Work out the finished part from the listing and answer in its coordinate system (mm). A direction names the side the tool comes from. Give positions to 0.01 mm unless a question says otherwise; leave off trailing zeros. Loops run counter-clockwise (first coordinate to the right, second up) from the corner with the lowest first, then second, coordinate; pieces in that order, holes last. Notation, with made-up numbers: (61.25, -3.5) - (115.25, -3.5) arc R25 ccw to (115.25, 8.5) - close; hole circle Ø9 at (40.25, 45). An arc over 180 degrees is marked (long way). One line per item, written item: value.
from build123d import *

# Parameters (mm, degrees)
SKETCH1_W           = 228.6
SKETCH1_H           = 339.725
BOSS_EXTRUDE1_DEPTH = 6.35
SKETCH2_W           = 6.35
SKETCH2_H           = 19.05
BOSS_EXTRUDE2_DEPTH = 25.4
FILLET1_R           = 9.525
FILLET2_R           = 8
SKETCH3_R           = 4.7625
CUT_EXTRUDE1_DEPTH  = 401.415210282
SKETCH5_R           = 3.175
CUT_EXTRUDE2_DEPTH  = 411.263568484
SKETCH9_W           = 145.328
SKETCH9_H           = 196.09
CUT_EXTRUDE3_DEPTH  = 411.263568484
FILLET3_R           = 25.4
FILLET4_R           = 6.35


with BuildPart() as part:
    # Sketch1 → Boss-Extrude1 (new body)
    with BuildSketch(Plane.XY):
        with Locations((114.3, -169.8625)):
            Rectangle(SKETCH1_W, SKETCH1_H)
    extrude(amount=BOSS_EXTRUDE1_DEPTH)

    # Sketch2 → Boss-Extrude2 (add)
    with BuildSketch(Plane.XY.offset(6.35)):
        with Locations((22.225, -35.56)):
            Rectangle(SKETCH2_W, SKETCH2_H)
        with Locations((47.879, -35.56)):
            Rectangle(SKETCH2_W, SKETCH2_H)
        with Locations((149.479, -35.56)):
            Rectangle(SKETCH2_W, SKETCH2_H)
        with Locations((175.133, -35.56)):
            Rectangle(SKETCH2_W, SKETCH2_H)
        with Locations((22.225, -304.8)):
            Rectangle(SKETCH2_W, SKETCH2_H)
        with Locations((47.879, -304.8)):
            Rectangle(SKETCH2_W, SKETCH2_H)
        with Locations((149.479, -304.8)):
            Rectangle(SKETCH2_W, SKETCH2_H)
        with Locations((175.133, -304.8)):
            Rectangle(SKETCH2_W, SKETCH2_H)
        with Locations((175.553, -132.588)):
            Rectangle(SKETCH2_W, SKETCH2_H)
        with Locations((206.287, -132.588)):
            Rectangle(SKETCH2_W, SKETCH2_H)
    extrude(amount=BOSS_EXTRUDE2_DEPTH)

    # Fillet1
    fillet1_edges = [part.edges().sort_by_distance(p)[0] for p in [
        (22.225, -314.325, 31.75),
        (22.225, -295.275, 31.75),
        (47.879, -314.325, 31.75),
        (47.879, -295.275, 31.75),
        (149.479, -314.325, 31.75),
        (149.479, -295.275, 31.75),
        (175.133, -314.325, 31.75),
        (175.133, -295.275, 31.75),
        (206.287, -142.113, 31.75),
        (206.287, -123.063, 31.75),
        (175.553, -142.113, 31.75),
        (175.553, -123.063, 31.75),
        (175.133, -45.085, 31.75),
        (175.133, -26.035, 31.75),
        (149.479, -45.085, 31.75),
        (149.479, -26.035, 31.75),
        (47.879, -45.085, 31.75),
        (47.879, -26.035, 31.75),
        (22.225, -45.085, 31.75),
        (22.225, -26.035, 31.75),
    ]]
    fillet(fillet1_edges, radius=FILLET1_R - 0.0001)  # a hair under: the kernel refuses the full size

    # Fillet2
    fillet2_edges = [part.edges().sort_by_distance(p)[0] for p in [
        (22.225, -295.275, 6.35),
        (19.05, -304.8, 6.35),
        (25.4, -304.8, 6.35),
        (22.225, -314.325, 6.35),
        (44.704, -304.8, 6.35),
        (47.879, -314.325, 6.35),
        (51.054, -304.8, 6.35),
        (47.879, -295.275, 6.35),
        (22.225, -26.035, 6.35),
        (19.05, -35.56, 6.35),
        (25.4, -35.56, 6.35),
        (22.225, -45.085, 6.35),
        (44.704, -35.56, 6.35),
        (47.879, -45.085, 6.35),
        (51.054, -35.56, 6.35),
        (47.879, -26.035, 6.35),
        (149.479, -26.035, 6.35),
        (146.304, -35.56, 6.35),
        (152.654, -35.56, 6.35),
        (149.479, -45.085, 6.35),
        (171.958, -35.56, 6.35),
        (175.133, -45.085, 6.35),
        (178.308, -35.56, 6.35),
        (175.133, -26.035, 6.35),
        (175.553, -123.063, 6.35),
        (172.378, -132.588, 6.35),
        (178.728, -132.588, 6.35),
        (175.553, -142.113, 6.35),
        (203.112, -132.588, 6.35),
        (206.287, -142.113, 6.35),
        (209.462, -132.588, 6.35),
        (206.287, -123.063, 6.35),
        (171.958, -304.8, 6.35),
        (175.133, -314.325, 6.35),
        (178.308, -304.8, 6.35),
        (175.133, -295.275, 6.35),
        (149.479, -295.275, 6.35),
        (146.304, -304.8, 6.35),
        (152.654, -304.8, 6.35),
        (149.479, -314.325, 6.35),
    ]]
    fillet(fillet2_edges, radius=FILLET2_R)

    # Sketch3 → Cut-Extrude1 (cut, through all)
    with BuildSketch(Plane.ZY.offset(-19.05)):
        with Locations(Location((22.225, -35.56, 0), (0, 0, 180))):
            Circle(SKETCH3_R)
        with Locations(Location((22.225, -132.588, 0), (0, 0, 180))):
            Circle(SKETCH3_R)
        with Locations(Location((22.225, -304.8, 0), (0, 0, 180))):
            Circle(SKETCH3_R)
    extrude(amount=-CUT_EXTRUDE1_DEPTH, mode=Mode.SUBTRACT)

    # Sketch5 → Cut-Extrude2 (cut, through all)
    with BuildSketch(Plane.XY.offset(6.35)):
        with Locations((12.7, -12.7)):
            Circle(SKETCH5_R)
        with Locations((34.925, -59.435)):
            Circle(SKETCH5_R)
        with Locations((131.954, -35.56)):
            Circle(SKETCH5_R)
        with Locations((215.9, -12.7)):
            Circle(SKETCH5_R)
        with Locations((162.306, -59.435)):
            Circle(SKETCH5_R)
        with Locations((190.92, -108.713)):
            Circle(SKETCH5_R)
        with Locations((158.028, -136.132936151)):
            Circle(SKETCH5_R)
        with Locations((190.92, -156.463)):
            Circle(SKETCH5_R)
        with Locations((215.9, -327.025)):
            Circle(SKETCH5_R)
        with Locations((162.306, -280.925)):
            Circle(SKETCH5_R)
        with Locations((131.954, -304.8)):
            Circle(SKETCH5_R)
        with Locations((65.404, -304.8)):
            Circle(SKETCH5_R)
        with Locations((35.052, -280.925)):
            Circle(SKETCH5_R)
        with Locations((12.7, -327.025)):
            Circle(SKETCH5_R)
    extrude(amount=-CUT_EXTRUDE2_DEPTH, mode=Mode.SUBTRACT)

    # Sketch9 → Cut-Extrude3 (cut, through all)
    with BuildSketch(Plane.XY.offset(6.35)):
        with Locations((72.664, -170.18)):
            Rectangle(SKETCH9_W, SKETCH9_H)
        Polygon((202.101108352, -255.525), (164.378, -194.009910842), (164.378, -255.525), align=None)
        Polygon((209.55, -181.863), (171.826891648, -181.863), (209.55, -243.378089158), align=None)
    extrude(amount=-CUT_EXTRUDE3_DEPTH, mode=Mode.SUBTRACT)

    # Fillet3
    fillet3_edges = [part.edges().sort_by_distance(p)[0] for p in [
        (145.328, -72.135, 3.175),
        (145.328, -268.225, 3.175),
        (0, -268.225, 3.175),
        (0, -72.135, 3.175),
    ]]
    fillet(fillet3_edges, radius=FILLET3_R)

    # Fillet4
    fillet4_edges = [part.edges().sort_by_distance(p)[0] for p in [
        (171.826891648, -181.863, 3.175),
        (209.55, -181.863, 3.175),
        (209.55, -243.378089158, 3.175),
        (164.378, -194.009910842, 3.175),
        (202.101108352, -255.525, 3.175),
        (164.378, -255.525, 3.175),
        (0, 0, 3.175),
        (228.6, 0, 3.175),
        (228.6, -339.725, 3.175),
        (0, -339.725, 3.175),
    ]]
    fillet(fillet4_edges, radius=FILLET4_R)


solid = part.part
1. Section A-A (y = -199) is taken. Write down the section's boundary in (x, z).
Output:
outline: (145.33, 0) - (182.34, 0) - (182.34, 6.35) - (145.33, 6.35) - close; (209.55, 0) - (228.6, 0) - (228.6, 6.35) - (209.55, 6.35) - close
2. Flat-ended cylindrical pins translate along their axes: pin 1 Ø3 at (x, z) = (150.5, 17.5) entering from -Y (3 decimals); pin 2 Ø3 at (x, z) = (21.5, 18.5) entering from +Y (3 decimals); pin 3 Ø5 at (y, z) = (-305, 25.5) entering from +X; pin 4 Ø12 at (x, z) = (162, 20.5) entering from -Y. Find the tip coordinate at first contact, or state that the pin passes through.
Output:
pin 1: stops at y = -314.325
pin 2: stops at y = -26.035
pin 3: stops at x = 178.31
pin 4: passes through
3. Find the intervals of material crossed by line 1 along X through (y, z) = (-31, 20.5); line 2 along Y through (x, z) = (109.5, 4) (3 decimals); line 3 along Y through (x, z) = (47, 18.5) (3 decimals), in increasing order.
Output:
line 1: x = 19.05 to 25.4, 44.7 to 51.05, 146.3 to 152.65, 171.96 to 178.31
line 2: y = -339.725 to -268.225, -72.135 to 0
line 3: y = -314.325 to -307.767, -301.833 to -295.275, -45.085 to -38.527, -32.593 to -26.035
4. For faces 1 (the flat face through (44.704, -31, 25)), 2 (the cylindrical face through (22.381, -291.791, 7.747)), 3 (the flat face through (149, -314.325, 18)), 4 (the flat face through (186.297, -229.752, 3.219)), 5 (the cylindrical face through (168.894, -132.343, 7.747)), determine the directions among +Z, -Z, +X, -X, +Y, -Y from which every point of the face is accessible in a straight line to the end or side of a thin tool.
Output:
face 1: +Z, +Y, -Y
face 2: +Z, +X, -X
face 3: +Z, +X, -X, -Y
face 4: +Z, -Z
face 5: +Z, -X
5. The mould has two halves that part along Z. Classify faces 6 (the cylindrical face through (149.435, -308.019, 25.735)), 7 (the flat face through (163, -167, 0)), 8 (the cylindrical face through (22.269, -311.609, 28.886)): released by +Z, released by -Z, zero draft, split by the parting line, or undercut.
Output:
face 6: undercut
face 7: released by -Z
face 8: released by +Z
